Part print with two shaded views. Sizes in mm from the minimum x, y, z corner. A direction names the side the tool comes from. Coordinates: 2 decimals unless noted, no trailing zeros. Write each loop counter-clockwise with the first axis right and the second up, starting at its lowest first coordinate (ties: lowest second). Pieces come first, ordered by that corner, then holes.
Q1. Which spindle directions (+Z, -Z, +X, -X, +Y, -Y) get a long thin tool onto all of the face, cutting with end or side? Do the marked faces 1, 2, 3, 4 and 5. Say none if no direction does.
Q2. Band-saw the part on C-C, the plane z = 3.5. Write the cut outline in (x, y).
Q3. Pin check, flat tips, straight feed: P1, Ø1, axis at y = 7, z = 4.5, coming from the -X side; P2, Ø4, axis at x = 16, z = 3, coming from the -Y side; P3, Ø2, axis at x = 7, z = 6, coming from the -Y side. Stop position of each tip, or through.
Q4. Band-saw the part on D-D, the plane y = 5. Write the cut outline in (x, z), plus the area to 3 significant figures.
Q5. Drill centre lines: probe 1 along Y at (x, z) = (25, 6.5); probe 2 along X at (y, z) = (17.25, 5.5) (3 decimals); probe 3 along Y at (x, z) = (2.25, 3.5). Where is each one in solid material? Low to high.
Q6. Band-saw the part on B-B, the plane x = 25. Write the cut outline in (y, z).
Q7. Pull direction X, two halves, no side cores. Call the marked faces 6, 7, 8 and 9: released by +X, released by -X, zero draft, split by the parting line, or undercut.
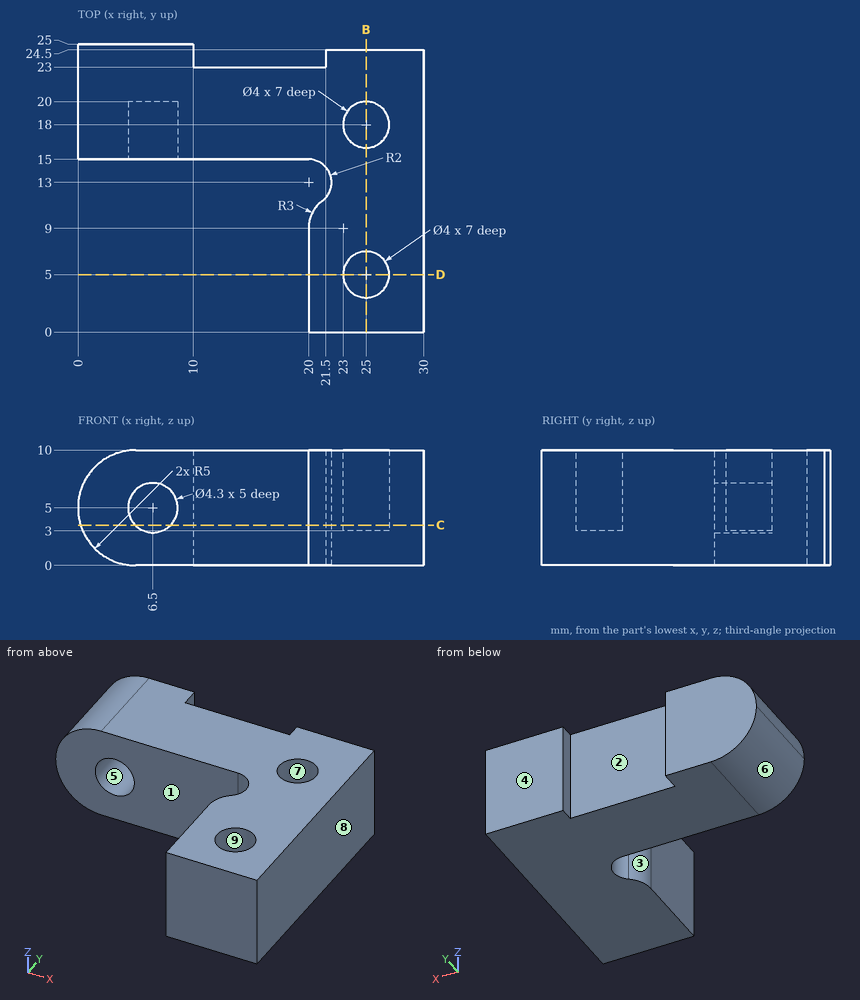
Answer sheet:
1. face 1: +Z, -Z, -X, -Y
1. face 2: +Z, -Z, +Y
1. face 3: +Z, -Z, -X
1. face 4: +Z, -Z, +X, +Y
1. face 5: -Y
2. outline: (0.23, 15) - (4.96, 15) - (4.96, 20) - (8.04, 20) - (8.04, 15) - (20, 15) arc R2 cw to (21.2, 11.4) arc R3 ccw to (20, 9) - (20, 0) - (30, 0) - (30, 24.5) - (21.5, 24.5) - (21.5, 23) - (10, 23) - (10, 25) - (0.23, 25) - close; hole circle Ø4 at (25, 5); hole circle Ø4 at (25, 18)
3. P1: stops at x = 20
3. P2: stops at y = 15
3. P3: stops at y = 20
4. outline: (20, 0) - (30, 0) - (30, 10) - (27, 10) - (27, 3) - (23, 3) - (23, 10) - (20, 10) - close
4. area: 72.0 mm2
5. probe 1: y = 0 to 3, 7 to 16, 20 to 24.5
5. probe 2: x = 0.025 to 4.409, 8.591 to 23.146, 26.854 to 30
5. probe 3: y = 15 to 25
6. outline: (0, 0) - (24.5, 0) - (24.5, 10) - (20, 10) - (20, 3) - (16, 3) - (16, 10) - (7, 10) - (7, 3) - (3, 3) - (3, 10) - (0, 10) - close
7. face 6: released by -X
7. face 7: undercut
7. face 8: released by +X
7. face 9: undercut
